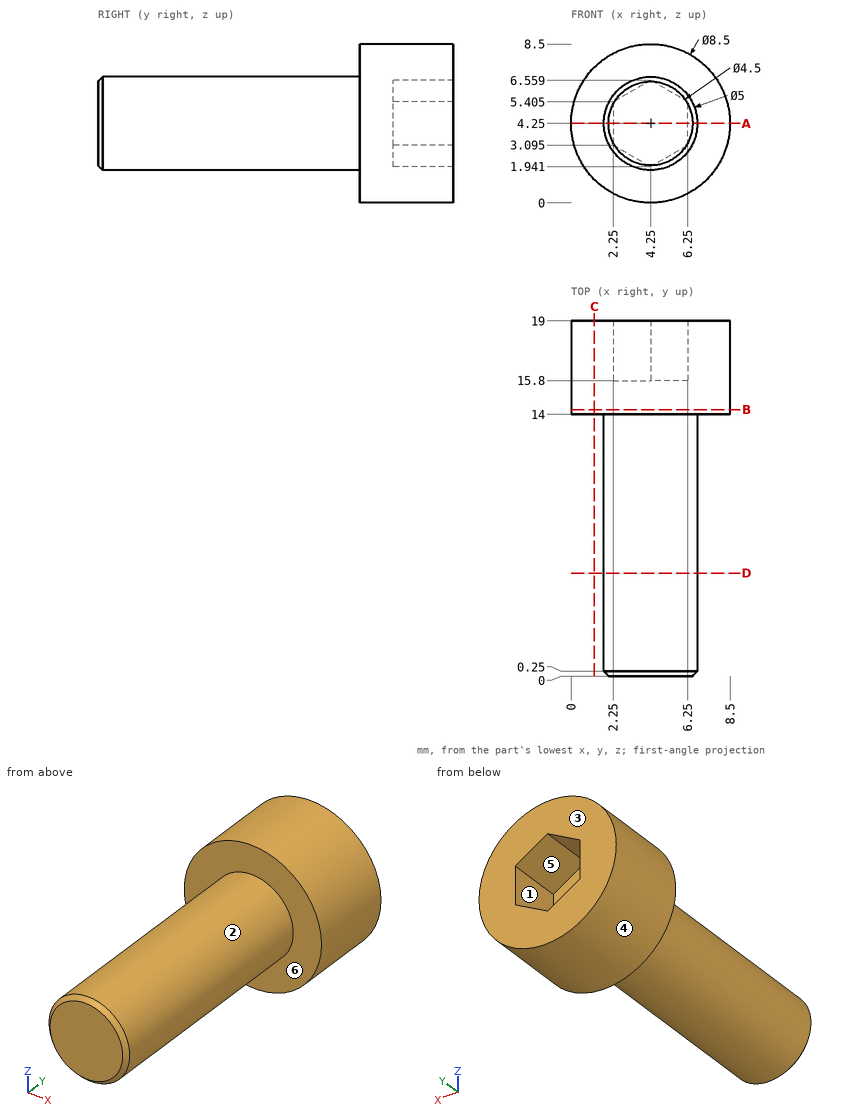
Can you work these out from the drawing? Everything is in mm from the part's minimum corner. A direction names the side the tool comes from. Round coordinates to 2 decimals unless told otherwise and drop trailing zeros. Order: outer loops, then holes, each group sorted by start corner. A loop starts at its lowest first (then second) coordinate and runs counter-clockwise, first axis right, second up. Notation, with made-up numbers: (7, 50) - (45, 50) arc R28 cw to (45, 70) - close; hole circle Ø6 at (-24.5, 68.5). An arc over 180 degrees is marked (long way). Answer in a Markdown table with one row per item.
(1) Suppose I cut it at B-B, the plane y = 14.25. Please give me the cut outline in (x, z).
From the geometry:
| item | result |
|---|---|
| outline | circle Ø8.5 at (4.25, 4.25) |
(2) If we mould it in two halves opening along Z, with no side actions, what happens to the marked faces 4, 5 and 6? For each: released by +Z, released by -Z, zero draft, split by the parting line, or undercut.
From the geometry:
| item | result |
|---|---|
| face 4 | split by the parting line |
| face 5 | undercut |
| face 6 | zero draft |
(3) Which directions (+Z, -Z, +X, -X, +Y, -Y) give clear straight access to the entire face, cutting with the end or side of a thin tool? Please do the marked faces 1, 2 and 3.
From the geometry:
| item | result |
|---|---|
| face 1 | +Y |
| face 2 | -Y |
| face 3 | +Z, -Z, +X, -X, +Y |
(4) Suppose I cut it at D-D, the plane y = 5.5. Please give me the cut outline in (x, z), plus the area to 3 significant figures.
From the geometry:
| item | result |
|---|---|
| outline | circle Ø5 at (4.25, 4.25) |
| area | 19.6 mm2 |
(5) Please list where these lines run through material, in increasing order: L1, parallel to Z at x = 2.75, y = 2; L2, parallel to Y at x = 6.75, z = 6.75; L3, parallel to X at y = 17.5, z = 5. Write a range as from..to.
From the geometry:
| item | result |
|---|---|
| L1 | z = 2.25..6.25 |
| L2 | y = 14..19 |
| L3 | x = 0.07..2.25, 6.25..8.43 |
(6) For P1, Ø3, axis at x = 2.5, y = 4, coming from the +Z side; P2, Ø1, axis at x = 4, y = 9.5, coming from the -Z side; P3, Ø3, axis at y = 11.5, z = 1, coming from the +X side (1 decimal), each with a flat end and sliding along its axis, tell me the tip position at first contact or that it passes through.
From the geometry:
| item | result |
|---|---|
| P1 | stops at z = 6.74 |
| P2 | stops at z = 1.75 |
| P3 | stops at x = 6 |
(7) Suppose I cut it at C-C, the plane x = 1.25. Please give me the cut outline in (y, z), plus the area to 3 significant figures.
From the geometry:
| item | result |
|---|---|
| outline | (14, 1.24) - (19, 1.24) - (19, 7.26) - (14, 7.26) - close |
| area | 30.1 mm2 |
(8) Suppose I cut it at A-A, the plane z = 4.25. Please give me the cut outline in (x, y).
From the geometry:
| item | result |
|---|---|
| outline | (0, 14) - (1.75, 14) - (1.75, 0.25) - (2, 0) - (6.5, 0) - (6.75, 0.25) - (6.75, 14) - (8.5, 14) - (8.5, 19) - (6.25, 19) - (6.25, 15.8) - (2.25, 15.8) - (2.25, 19) - (0, 19) - close |
